```python
from build123d import *

# Parameters (mm, degrees)
SKETCH1_W           = 85
SKETCH1_H           = 72
BOSS_EXTRUDE1_DEPTH = 98
SKETCH2_R           = 4
CUT_EXTRUDE1_DEPTH  = 10
SKETCH3_R           = 6
BOSS_EXTRUDE2_DEPTH = 30


with BuildPart() as part:
    # Sketch1 → Boss-Extrude1 (new body)
    with BuildSketch(Plane(origin=(0, 0, 0), x_dir=(1, 0, 0), z_dir=(0, 1, 0))):
        Rectangle(SKETCH1_W, SKETCH1_H)
    extrude(amount=BOSS_EXTRUDE1_DEPTH)

    # Sketch2 → Cut-Extrude1 (cut)
    with BuildSketch(Plane(origin=(0, 98, 0), x_dir=(1, 0, 0), z_dir=(0, 1, 0))):
        with Locations(Location((0, 3.5, 0), (0, 0, 270))):
            Circle(SKETCH2_R)
    extrude(amount=-CUT_EXTRUDE1_DEPTH, mode=Mode.SUBTRACT)

    # Sketch3 → Boss-Extrude2 (add)
    with BuildSketch(Plane.XY.offset(36)):
        with Locations(Location((0, 43, 0), (0, 0, 180))):
            Circle(SKETCH3_R)
    extrude(amount=BOSS_EXTRUDE2_DEPTH)


solid = part.part
```
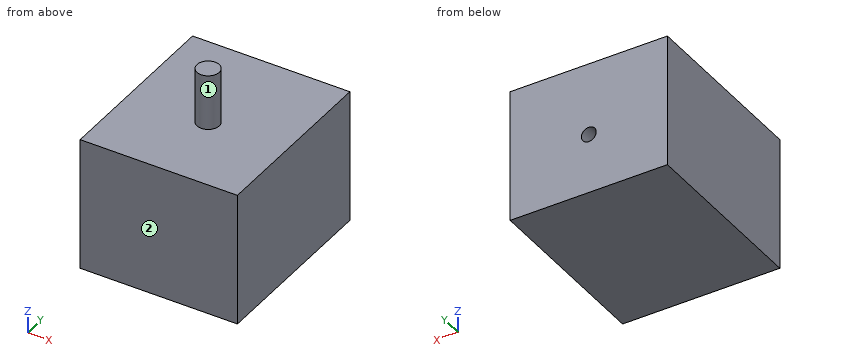
Geometry check sheet. Reference: the model listing, model coordinates, mm. Face numbers are marked on the shaded views. A direction names the side the tool comes from. Round coordinates to 2 decimals unless told otherwise and drop trailing zeros. Order: outer loops, then holes, each group sorted by start corner. A loop starts at its lowest first (then second) coordinate and runs counter-clockwise, first axis right, second up. Notation, with made-up numbers: (-12.75, -19.75) - (14.25, -19.75) arc R27 cw to (14.25, 16.25) - close; hole circle Ø10 at (-9, 75). An arc over 180 degrees is marked (long way). Use a Markdown table: item, result. Add a question column.
1) Section check D-D (x = -12). Record the cut outline in (y, z), then the cut area to 3 significant figures.
2) Section check C-C (z = 51). Record the cut outline in (x, y).
3) Section check A-A (x = 0). Record the cut outline in (y, z).
4) Set-up check for the marked faces 1 and 2: record each of +Z, -Z, +X, -X, +Y, -Y from which the full face is reachable in a straight line by a thin tool's end or side.
5) Section check B-B (y = 43). Record the cut outline in (x, z).
6) Thickness scan on line 1 along X through (y, z) = (94, -3); line 2 along Z through (x, y) = (-1, 51). Record the ranges inside material, lowest first.
7) Gauge pin test, flat ends, axial feed: P1, Ø2.5, axis at x = -1.5, z = -4.5, coming from the +Y side; P2, Ø5, axis at x = -26.5, y = 72, coming from the +Z side. Record the tip position at first contact, or that the pin passes through.
Established:
| question | item | result |
|---|---|---|
| 1 | outline | (0, -36) - (98, -36) - (98, 36) - (0, 36) - close |
| 1 | area | 7,060 mm2 |
| 2 | outline | circle Ø12 at (0, 43) |
| 3 | outline | (0, -36) - (98, -36) - (98, -7.5) - (88, -7.5) - (88, 0.5) - (98, 0.5) - (98, 36) - (49, 36) - (49, 66) - (37, 66) - (37, 36) - (0, 36) - close |
| 4 | face 1 | +Z |
| 4 | face 2 | +Z, -Z, +X, -X, -Y |
| 5 | outline | (-42.5, -36) - (42.5, -36) - (42.5, 36) - (6, 36) - (6, 66) - (-6, 66) - (-6, 36) - (-42.5, 36) - close |
| 6 | line 1 | -42.5 to -3.97, 3.97 to 42.5 |
| 6 | line 2 | -36 to 36 |
| 7 | P1 | y = 88 |
| 7 | P2 | z = 36 |
